Can you work these out from the model? Positions are in its coordinate system, mm. Give positions to 0.01 mm unless a question says otherwise; leave off trailing zeros. Write each loop counter-clockwise with the first axis right and the second up, starting at its lowest first coordinate (ties: lowest second). Pieces come first, ordered by that corner, then holes.
from build123d import *

# Parameters (mm, degrees)
SKETCH1_W                = 30
SKETCH1_H                = 30
BOSS_EXTRUDE1_DEPTH      = 332.5
BOSS_EXTRUDE1_DEPTH_BACK = 332.5
SKETCH2_W                = 30
SKETCH2_H                = 30
BOSS_EXTRUDE2_DEPTH      = 700


with BuildPart() as part:
    # Sketch1 → Boss-Extrude1 (new body, two sides)
    with BuildSketch(Plane(origin=(0, 0, 0), x_dir=(0, 0, -1), z_dir=(1, 0, 0))) as boss_extrude1_sk:
        Rectangle(SKETCH1_W, SKETCH1_H)
    extrude(amount=BOSS_EXTRUDE1_DEPTH)
    extrude(boss_extrude1_sk.sketch, amount=-BOSS_EXTRUDE1_DEPTH_BACK)

    # Sketch2 → Boss-Extrude2 (add)
    with BuildSketch(Plane(origin=(0, 0, 0), x_dir=(-1, 0, 0), z_dir=(0, -0.970295726, 0.241921896))):
        Rectangle(SKETCH2_W, SKETCH2_H)
    extrude(amount=BOSS_EXTRUDE2_DEPTH)


solid = part.part
(1) Imagine slicing it at B-B, the plane z = -3. Write out the boundary of the cut face in (x, y).
Returned:
outline: (-332.5, -15) - (-15, -15) - (-15, -49.97) - (15, -49.97) - (15, -15) - (332.5, -15) - (332.5, 15) - (-332.5, 15) - close
(2) Imagine slicing it at A-A, the plane x = 292. Write out the boundary of the cut face in (y, z), plus the area to 3 significant figures.
Returned:
outline: (-15, -15) - (15, -15) - (15, 15) - (-15, 15) - close
area: 900 mm2
(3) If I drill on L1, parallel to X at y = -575.5, z = 132.5, over which ranges is the centre line in solid material (lowest first)?
Returned:
L1: x = -15 to 15
(4) Imagine slicing it at C-C, the plane y = -429. Write out the boundary of the cut face in (x, z).
Returned:
outline: (-15, 91.5) - (15, 91.5) - (15, 122.42) - (-15, 122.42) - close
(5) Will these pins go through, and if not, where does the flat tip stop? P1, Ø2, axis at x = 5.5, y = -202, coming from the +Z side; P2, Ø10, axis at x = -18.5, y = -554, coming from the -Z side; P3, Ø1.5, axis at y = -416.5, z = 94.5, coming from the +X side.
Returned:
P1: stops at z = 66.07
P2: stops at z = 121.78
P3: stops at x = 15
